Could you check a few things on this model? Use its own coordinates, in mm. Face numbers are marked on the shaded views. A direction names the side the tool comes from. Round coordinates to 2 decimals unless told otherwise and drop trailing zeros. Order: outer loops, then holes, each group sorted by start corner. A loop starts at its lowest first (then second) coordinate and runs counter-clockwise, first axis right, second up. Notation, with made-up numbers: (3, 39.25) -> (31, 39.25) arc R14 ccw to (31, 62.25) -> close; hole circle Ø7 at (14.25, 67.5). An arc over 180 degrees is marked (long way). One line per question, with ' | ' between items.
```python
from build123d import *

# Parameters (mm, degrees)
SKETCH001_W      = 8.45
SKETCH001_H      = 8.45
EXTRUDE001_DEPTH = 3
SKETCH_W         = 54.25
SKETCH_H         = 12.5
SKETCH_W_2       = 8.45
SKETCH_H_2       = 8.45
EXTRUDE_DEPTH    = 6.8


with BuildPart() as extrude001:
    # Sketch001 → Extrude001 (new body)
    with BuildSketch(Plane.XY):
        with Locations((-45.5, 0)):
            Rectangle(SKETCH001_W, SKETCH001_H)
        with Locations((8, 0)):
            Rectangle(SKETCH001_W, SKETCH001_H)
    extrude(amount=EXTRUDE001_DEPTH)


with BuildPart() as cut:
    # Sketch → Extrude (new body)
    with BuildSketch(Plane.XY):
        with Locations((-20.9, -0.025)):
            Rectangle(SKETCH_W, SKETCH_H)
        Rectangle(SKETCH_W_2, SKETCH_H_2, mode=Mode.SUBTRACT)
        with Locations((-10.45, 0)):
            Rectangle(SKETCH_W_2, SKETCH_H_2, mode=Mode.SUBTRACT)
        with Locations((-20.9, 0)):
            Rectangle(SKETCH_W_2, SKETCH_H_2, mode=Mode.SUBTRACT)
        with Locations((-31.35, 0)):
            Rectangle(SKETCH_W_2, SKETCH_H_2, mode=Mode.SUBTRACT)
        with Locations((-41.8, 0)):
            Rectangle(SKETCH_W_2, SKETCH_H_2, mode=Mode.SUBTRACT)
    extrude(amount=EXTRUDE_DEPTH)

    # Cut: cut Extrude001
    add(extrude001.part, mode=Mode.SUBTRACT)


solid = cut.part
```
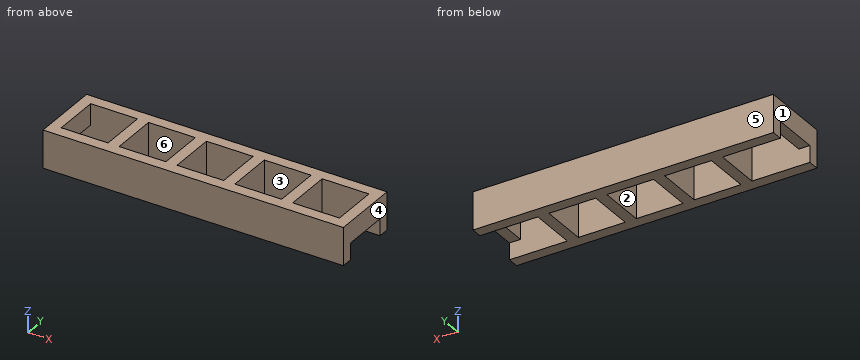
1. If we mould it in two halves opening along X, with no side actions, what happens to the marked faces 3, 4, 5 and 6? For each: pulls with the +X half, pulls with the -X half, needs draft (parallel to the pull), parting line crosses it, or undercut.
From the geometry:
face 3: undercut | face 4: pulls with the +X half | face 5: needs draft | face 6: undercut
2. I want a section at D-D on z = 1.5. List the corners of the cut face in (x, y) for me (3 decimals).
From the geometry:
outline: (-48.025, -6.275) -> (6.225, -6.275) -> (6.225, -4.225) -> (-4.225, -4.225) -> (-4.225, 4.225) -> (6.225, 4.225) -> (6.225, 6.225) -> (-48.025, 6.225) -> (-48.025, 4.225) -> (-37.575, 4.225) -> (-37.575, -4.225) -> (-48.025, -4.225) -> close; hole (-35.575, -4.225) -> (-27.125, -4.225) -> (-27.125, 4.225) -> (-35.575, 4.225) -> close; hole (-25.125, -4.225) -> (-16.675, -4.225) -> (-16.675, 4.225) -> (-25.125, 4.225) -> close; hole (-14.675, -4.225) -> (-6.225, -4.225) -> (-6.225, 4.225) -> (-14.675, 4.225) -> close
3. I'm going to push flat-ended pins straight in: pin 1 (1.6 mm diameter, centred on x = -46.5, y = 1.5, fed in from -Z); pin 2 (1.5 mm diameter, centred on x = -28, y = -1.5, fed in from -Z). Where does each tip first touch, or does it pass through?
From the geometry:
pin 1: stops at z = 3 | pin 2: passes through
4. On a 3-axis mill with a long thin cutter (end or side, diameter ignored), from which of +Z, -Z, +X, -X, +Y, -Y can I reach the whole of each face in a straight line? I mean the marked faces 1 and 2. Say none if no direction works.
From the geometry:
face 1: +Z, -Z, -X, +Y, -Y | face 2: +Z, -Z
5. I want a section at C-C on x = -24. List the corners of the cut face in (y, z) for me (3 decimals), and give its area (3 significant figures).
From the geometry:
outline: (-6.275, 0) -> (-4.225, 0) -> (-4.225, 6.8) -> (-6.275, 6.8) -> close; (4.225, 0) -> (6.225, 0) -> (6.225, 6.8) -> (4.225, 6.8) -> close | area: 27.5 mm²
6. I need wall thicknesses on probe 1 along X at (y, z) = (-2.25, 2) (3 decimals); probe 2 along X at (y, z) = (2.5, 5.25) (3 decimals); probe 3 along Y at (x, z) = (-28.5, 3.75) (3 decimals). Which ranges of each line are inside material? Lowest first, please.
From the geometry:
probe 1: x = -37.575 to -35.575, -27.125 to -25.125, -16.675 to -14.675, -6.225 to -4.225 | probe 2: x = -48.025 to -46.025, -37.575 to -35.575, -27.125 to -25.125, -16.675 to -14.675, -6.225 to -4.225, 4.225 to 6.225 | probe 3: y = -6.275 to -4.225, 4.225 to 6.225
7. I want a section at A-A on y = 1.75. List the corners of the cut face in (x, z) for me (3 decimals), and give its area (3 significant figures).
From the geometry:
outline: (-48.025, 3) -> (-46.025, 3) -> (-46.025, 6.8) -> (-48.025, 6.8) -> close; (-37.575, 0) -> (-35.575, 0) -> (-35.575, 6.8) -> (-37.575, 6.8) -> close; (-27.125, 0) -> (-25.125, 0) -> (-25.125, 6.8) -> (-27.125, 6.8) -> close; (-16.675, 0) -> (-14.675, 0) -> (-14.675, 6.8) -> (-16.675, 6.8) -> close; (-6.225, 0) -> (-4.225, 0) -> (-4.225, 6.8) -> (-6.225, 6.8) -> close; (4.225, 3) -> (6.225, 3) -> (6.225, 6.8) -> (4.225, 6.8) -> close | area: 69.6 mm²
8. I want a section at B-B on z = 6. List the corners of the cut face in (x, y) for me (3 decimals).
From the geometry:
outline: (-48.025, -6.275) -> (6.225, -6.275) -> (6.225, 6.225) -> (-48.025, 6.225) -> close; hole (-46.025, -4.225) -> (-37.575, -4.225) -> (-37.575, 4.225) -> (-46.025, 4.225) -> close; hole (-35.575, -4.225) -> (-27.125, -4.225) -> (-27.125, 4.225) -> (-35.575, 4.225) -> close; hole (-25.125, -4.225) -> (-16.675, -4.225) -> (-16.675, 4.225) -> (-25.125, 4.225) -> close; hole (-14.675, -4.225) -> (-6.225, -4.225) -> (-6.225, 4.225) -> (-14.675, 4.225) -> close; hole (-4.225, -4.225) -> (4.225, -4.225) -> (4.225, 4.225) -> (-4.225, 4.225) -> close
